Geometry check sheet. Reference: the model listing, model coordinates, mm. Face numbers are marked on the shaded views. Coordinates: 2 decimals unless noted, no trailing zeros. Write each loop counter-clockwise with the first axis right and the second up, starting at its lowest first coordinate (ties: lowest second). Pieces come first, ordered by that corner, then holes. Notation, with made-up numbers: (-39, 74.25) -> (16, 74.25) arc R28 cw to (16, 95.25) -> close; hole circle Ø3 at (35.25, 73.25). An arc over 180 degrees is marked (long way). Use a Markdown table: item, result.
```python
from build123d import *

# Parameters (mm, degrees)
SKETCH1_R                = 20
BOSS_EXTRUDE1_DEPTH      = 3.5
SKETCH2_R                = 35
SKETCH2_R_2              = 20
SKETCH2_R_3              = 2.8
BOSS_EXTRUDE2_DEPTH      = 8
BOSS_EXTRUDE3_DEPTH      = 2
BOSS_EXTRUDE3_DEPTH_BACK = 8
SKETCH4_R                = 2.9
SKETCH5_R                = 5
BOSS_EXTRUDE4_DEPTH      = 3
CUT_EXTRUDE1_START       = -10
SKETCH3_R                = 20
CUT_EXTRUDE1_DEPTH       = 10
SKETCH9_R                = 18.5
BOSS_EXTRUDE5_DEPTH      = 3.5
SKETCH10_R               = 18.5
SKETCH10_R_2             = 17.5
BOSS_EXTRUDE6_DEPTH      = 3.5
SKETCH11_W               = 2
SKETCH11_H               = 6.599117057
BOSS_EXTRUDE7_DEPTH      = 2
SKETCH12_R               = 72.135852014
CUT_EXTRUDE2_DEPTH       = 22
FILLET1_R                = 10
CUT_EXTRUDE3_START       = -10
SKETCH13_R               = 20
CUT_EXTRUDE3_DEPTH       = 10


with BuildPart() as part:
    # Sketch1 → Boss-Extrude1 (new body)
    with BuildSketch(Plane(origin=(0, 0, 0), x_dir=(1, 0, 0), z_dir=(0, 1, 0))):
        with Locations(Location((0, 0, 0), (0, 0, 270))):
            Circle(SKETCH1_R)
    extrude(amount=BOSS_EXTRUDE1_DEPTH)

    # Sketch2 → Boss-Extrude2 (add)
    with BuildSketch(Plane(origin=(0, 0, 0), x_dir=(1, 0, 0), z_dir=(0, 1, 0))):
        with Locations(Location((0, 0, 0), (0, 0, 270))):
            Circle(SKETCH2_R)
        with Locations(Location((0, 0, 0), (0, 0, 270))):
            Circle(SKETCH2_R_2, mode=Mode.SUBTRACT)
        with Locations(Location((0, 29, 0), (0, 0, 270))):
            Circle(SKETCH2_R_3, mode=Mode.SUBTRACT)
        with Locations(Location((25.11473671, -14.5, 0), (0, 0, 270))):
            Circle(SKETCH2_R_3, mode=Mode.SUBTRACT)
        with Locations(Location((-25.11473671, -14.5, 0), (0, 0, 270))):
            Circle(SKETCH2_R_3, mode=Mode.SUBTRACT)
    extrude(amount=BOSS_EXTRUDE2_DEPTH)

    # Sketch4 → Boss-Extrude3 (add, two sides: drawn at the far end of the back side and taken through both)
    with BuildSketch(Plane.XZ.offset(-BOSS_EXTRUDE3_DEPTH_BACK)):
        with Locations(Location((-25.11473671, 14.5, 0), (0, 0, 270))):
            Circle(SKETCH4_R)
        with Locations(Location((25.11473671, 14.5, 0), (0, 0, 270))):
            Circle(SKETCH4_R)
        with Locations(Location((0, -29, 0), (0, 0, 270))):
            Circle(SKETCH4_R)
    extrude(amount=BOSS_EXTRUDE3_DEPTH + BOSS_EXTRUDE3_DEPTH_BACK)

    # Sketch5 → Boss-Extrude4 (add)
    with BuildSketch(Plane(origin=(0, 8, 0), x_dir=(1, 0, 0), z_dir=(0, 1, 0))):
        with Locations((-30.453629482, -17.250404383)):
            Circle(SKETCH5_R)
        with Locations((0.28752632, 34.99881896)):
            Circle(SKETCH5_R)
        with Locations((30.166103162, -17.748414577)):
            Circle(SKETCH5_R)
    extrude(amount=-BOSS_EXTRUDE4_DEPTH)

    # Sketch3 → Cut-Extrude1 (cut)
    with BuildSketch(Plane(origin=(0, 3.5, 0), x_dir=(1, 0, 0), z_dir=(0, 1, 0)).offset(CUT_EXTRUDE1_START)):
        with Locations(Location((0, 0, 0), (0, 0, 270))):
            Circle(SKETCH3_R)
    extrude(amount=CUT_EXTRUDE1_DEPTH, mode=Mode.SUBTRACT)



with BuildPart() as body_2:
    # Sketch9 → Boss-Extrude5 (new body)
    with BuildSketch(Plane(origin=(0, 8, 0), x_dir=(1, 0, 0), z_dir=(0, 1, 0))):
        with Locations(Location((0, 0, 0), (0, 0, 270))):
            Circle(SKETCH9_R)
    extrude(amount=-BOSS_EXTRUDE5_DEPTH)

    # Sketch10 → Boss-Extrude6 (add)
    with BuildSketch(Plane(origin=(0, 4.5, 0), x_dir=(-1, 0, 0), z_dir=(0, -1, 0))):
        with Locations(Location((0, 0, 0), (0, 0, 270))):
            Circle(SKETCH10_R)
        with Locations(Location((0, 0, 0), (0, 0, 90))):
            Circle(SKETCH10_R_2, mode=Mode.SUBTRACT)
    extrude(amount=BOSS_EXTRUDE6_DEPTH)


with BuildPart() as part_1:
    add(part.part)

    add(body_2.part)  # Boss-Extrude7 merges body 2
    # Sketch11 → Boss-Extrude7 (add)
    with BuildSketch(Plane(origin=(0, 8, 0), x_dir=(1, 0, 0), z_dir=(0, 1, 0))):
        Polygon((19.946286756, -10.36129349), (14.231283742, -7.061734961), (13.231283742, -8.793785769), (18.946286756, -12.093344297), align=None)
        with Locations((0, 19.155079259)):
            Rectangle(SKETCH11_W, SKETCH11_H)
        Polygon((-18.946286756, -12.093344297), (-13.231283742, -8.793785769), (-14.231283742, -7.061734961), (-19.946286756, -10.36129349), align=None)
    extrude(amount=-BOSS_EXTRUDE7_DEPTH)

    # Sketch12 → Cut-Extrude2 (cut)
    with BuildSketch(Plane(origin=(0, 8, 0), x_dir=(1, 0, 0), z_dir=(0, 1, 0))):
        Circle(SKETCH12_R)
        Polygon((0, 52), (-45.033320997, -26), (45.033320997, -26), align=None, mode=Mode.SUBTRACT)
    extrude(amount=-CUT_EXTRUDE2_DEPTH, mode=Mode.SUBTRACT)

    # Fillet1
    fillet1_edges = [part_1.edges().sort_by_distance(p)[0] for p in [
        (34.232035012, 4, 7.291623888),
        (10.801285985, 4, -33.291623888),
        (-23.430749028, 4, 26),
        (23.430749028, 4, 26),
        (-10.801285985, 4, -33.291623888),
        (-34.232035012, 4, 7.291623888),
    ]]
    fillet(fillet1_edges, radius=FILLET1_R)

    # Sketch13 → Cut-Extrude3 (cut)
    with BuildSketch(Plane(origin=(0, 8, 0), x_dir=(1, 0, 0), z_dir=(0, 1, 0)).offset(CUT_EXTRUDE3_START)):
        with Locations(Location((0, 0, 0), (0, 0, 270))):
            Circle(SKETCH13_R)
    extrude(amount=CUT_EXTRUDE3_DEPTH, mode=Mode.SUBTRACT)


solid = part_1.part
```
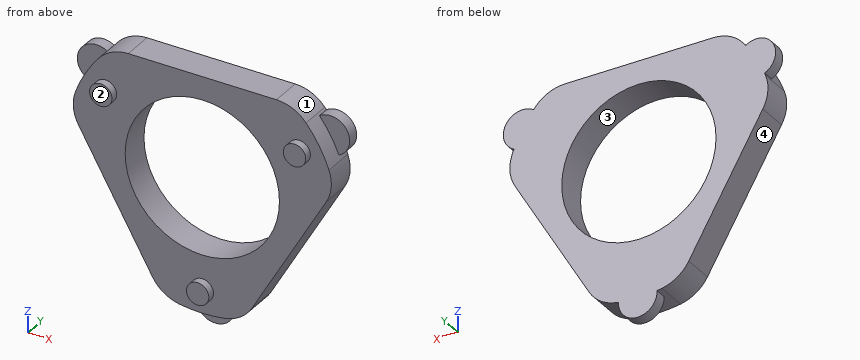
Item 1: Section check C-C on y = 7. Record the boundary of the cut face in (x, z), then the cut area to 3 significant figures.
Answer block:
| item | result |
|---|---|
| outline | (-32.85, 12.09) arc R10 ccw to (-32.12, 3.64) -> (-12.91, -29.64) arc R10 ccw to (-5.95, -34.49) arc R35 ccw to (-4.7, -34.68) arc R5 ccw (long way) to (5.27, -34.6) arc R35 ccw to (5.95, -34.49) arc R10 ccw to (12.91, -29.64) -> (32.12, 3.64) arc R10 ccw to (32.85, 12.09) arc R35 ccw to (32.39, 13.27) arc R5 ccw (long way) to (27.33, 21.87) arc R35 ccw to (26.89, 22.4) arc R10 ccw to (19.21, 26) -> (-19.21, 26) arc R10 ccw to (-26.89, 22.4) arc R35 ccw to (-27.68, 21.41) arc R5 ccw (long way) to (-32.6, 12.73) arc R35 ccw to start; hole circle Ø40 at (0, 0) |
| area | 1,830 mm^2 |
Item 2: Section check D-D on z = 14.5. Record the boundary of the cut face in (x, y), then the cut area to 3 significant figures.
Answer block:
| item | result |
|---|---|
| outline | (-34.63, 5) -> (-31.86, 5) -> (-31.86, 0) -> (-28.01, 0) -> (-28.01, -2) -> (-22.21, -2) -> (-22.21, 0) -> (-13.77, 0) -> (-13.77, 8) -> (-34.63, 8) -> close; (13.77, 0) -> (22.21, 0) -> (22.21, -2) -> (28.01, -2) -> (28.01, 0) -> (31.86, 0) -> (31.86, 5) -> (33.97, 5) -> (33.97, 8) -> (13.77, 8) -> close |
| area | 327 mm^2 |
Item 3: Mould release check, pull along Z, two halves, no side actions. Record for the marked faces 1, 2, 3 and 4: +Z half, -Z half, draft (parallel to the pull), parting line (faces both ways), or undercut.
Answer block:
| item | result |
|---|---|
| face 1 | +Z half |
| face 2 | draft |
| face 3 | undercut |
| face 4 | -Z half |
Item 4: Section check B-B on x = -8.5. Record the boundary of the cut face in (y, z), then the cut area to 3 significant figures.
Answer block:
| item | result |
|---|---|
| outline | (0, -33.69) -> (8, -33.69) -> (8, -18.1) -> (0, -18.1) -> close; (0, 18.1) -> (8, 18.1) -> (8, 26) -> (0, 26) -> close |
| area | 188 mm^2 |
Item 5: Section check A-A on z = 0.5. Record the boundary of the cut face in (x, y).
Answer block:
| item | result |
|---|---|
| outline | (-30.31, 0) -> (-19.99, 0) -> (-19.99, 8) -> (-30.31, 8) -> close; (19.99, 0) -> (30.31, 0) -> (30.31, 8) -> (19.99, 8) -> close |
Item 6: Thickness scan on L1, parallel to Z at x = 0, y = 3; L2, parallel to Z at x = 0, y = 5.75; L3, parallel to Y at x = -9, z = -18. Record the ranges inside material, lowest first. Write a range as [from, to].
Answer block:
| item | result |
|---|---|
| L1 | z = [-35, -20], [20, 26] |
| L2 | z = [-39.99, -20], [20, 26] |
| L3 | y = [0, 8] |
Item 7: Depth check by flat-ended pin: P1, Ø2.5, axis at x = -30, z = 19, coming from the -Y side; P2, Ø3, axis at y = 3, z = 18.5, coming from the -X side; P3, Ø1, axis at y = 5, z = -23.5, coming from the +X side. Enter the tip coordinate at first touch or a pass-through.
Answer block:
| item | result |
|---|---|
| P1 | stops at y = 0 |
| P2 | stops at x = -30.59 |
| P3 | stops at x = 16.74 |
